Build history of the part. All positions in model axes, mm. A direction names the side the tool comes from. Coordinates: 2 decimals unless noted, no trailing zeros. Loops run counter-clockwise (first coordinate to the right, second up) from the corner with the lowest first, then second, coordinate; pieces in that order, holes last.
Item 1: 3-axis set-ups, long thin cutter, end or side, ignore diameter. For faces 1 (the face through (-32.5, 1, -71)), 2 (the face through (32.5, 1, -4)), 3 (the face through (-18, 2, 76)), 4 (the face through (32.5, 1, -71)): which of +Z, -Z, +X, -X, +Y, -Y reach the whole face in a straight line?
Item 2: Flat gauge pins, fed straight in: pin 1 (0.9 mm diameter, centred on y = 1, z = 60, fed in from -X); pin 2 (1.5 mm diameter, centred on x = 28, y = 1, fed in from +Z); pin 3 (0.8 mm diameter, centred on x = -33, y = 1, fed in from -Z). Where does each tip first touch, or does it go through?
Item 3: Drill centre lines: line 1 along Z through (x, y) = (-15.5, 1.9); line 2 along Y through (x, z) = (-3, -30.5); line 3 along X through (y, z) = (1.4, -46). Where is each one in solid material? Low to high.
Item 4: Cut at B-B (z = -51.5). List the corners of the cut face in (x, y), and give its area (3 significant figures).
Item 5: Mould opens along Z. For faces 5 (the face through (29, 2, 76)), 6 (the face through (-32.5, 1, -4)), 7 (the face through (-1, 0, 1)) say: released by +Z, released by -Z, zero draft, split by the parting line, or undercut.
from build123d import *

# Parameters (mm, degrees)
CROQUIS1_W               = 65
CROQUIS1_H               = 146
SALIENTE_EXTRUIR1_DEPTH  = 3
CROQUIS2_W               = 8
CROQUIS2_H               = 3
SALIENTE_EXTRUIR2_DEPTH  = 5
REDONDEO1_R              = 4
REDONDEO1_OF_SIMETR_A1_R = 4
CROQUIS3_W               = 2.60095456
CROQUIS3_H               = 3.001101416
SALIENTE_EXTRUIR3_DEPTH  = 0.8
REDONDEO2_R              = 2
REDONDEO2_OF_SIMETR_A5_R = 2
CROQUIS4_W               = 65
CROQUIS4_H               = 3
CROQUIS4_W_2             = 30
CROQUIS4_H_2             = 2
SALIENTE_EXTRUIR4_DEPTH  = 3
REDONDEO3_R              = 60


# Some blends are built 0.0001 mm under size
with BuildPart() as part:
    # Croquis1 → Saliente-Extruir1 (new body)
    with BuildSketch(Plane(origin=(0, 0, 0), x_dir=(1, 0, 0), z_dir=(0, 1, 0))):
        Rectangle(CROQUIS1_W, CROQUIS1_H)
    extrude(amount=SALIENTE_EXTRUIR1_DEPTH)

    # Croquis2 → Saliente-Extruir2 (add)
    with BuildSketch(Plane(origin=(32.5, 0, 0), x_dir=(0, 0, -1), z_dir=(1, 0, 0))):
        with Locations((66, 1.5)):
            Rectangle(CROQUIS2_W, CROQUIS2_H)
    saliente_extruir2 = extrude(amount=SALIENTE_EXTRUIR2_DEPTH)

    # Redondeo1
    redondeo1_edges = [part.edges().sort_by_distance(p)[0] for p in [
        (37.5, 1.5, -62),
        (37.5, 1.5, -70),
    ]]
    fillet(redondeo1_edges, radius=REDONDEO1_R - 0.0001)  # a hair under: the kernel refuses the full size

    # Simetría1: Saliente-Extruir2 across plane
    add(saliente_extruir2.mirror(Plane(origin=(0, 0, 0), x_dir=(0, 0, 1), z_dir=(1, 0, 0))))

    # Redondeo1 of Simetría1
    redondeo1_of_simetr_a1_edges = [part.edges().sort_by_distance(p)[0] for p in [
        (-37.5, 1.5, -62),
        (-37.5, 1.5, -70),
    ]]
    fillet(redondeo1_of_simetr_a1_edges, radius=REDONDEO1_OF_SIMETR_A1_R - 0.0001)  # a hair under: the kernel refuses the full size

    # Croquis3 → Saliente-Extruir3 (add)
    with BuildSketch(Plane(origin=(32.5, 0, 0), x_dir=(0, 0, -1), z_dir=(1, 0, 0))):
        with Locations((-53.003039433, 1.500550708)):
            Rectangle(CROQUIS3_W, CROQUIS3_H)
    saliente_extruir3 = extrude(amount=SALIENTE_EXTRUIR3_DEPTH)

    # Redondeo2
    # the kernel refuses this fillet: 2 mm, written as the material it takes off along each edge
    with BuildSketch(Plane(origin=(33.3, 7.001101416, 51.702562153), x_dir=(-1, 0, 0), z_dir=(0, -1, 0)), Plane(origin=(33.3, -4, 54.303516713), x_dir=(-1, 0, 0), z_dir=(0, 1, 0))) as redondeo2_piece_1:
        with BuildLine():
            CenterArc((2, -1.6), REDONDEO2_R, 126.869897646, 53.130102354)
            Line((0, -1.6), (-0.04, -1.6))
            Line((-0.04, -1.6), (-0.04, 0))
            Line((-0.04, 0), (0, 0.04))
            ThreePointArc((0, 0.04), (0.4, 0.04), (0.776, 0.032))
            Line((0.776, 0.032), (0.8, 0))
        make_face()
    extrude(amount=11.001101416, mode=Mode.SUBTRACT)

    # Simetría5: Saliente-Extruir3 across plane
    add(saliente_extruir3.mirror(Plane(origin=(0, 0, 0), x_dir=(0, 0, 1), z_dir=(1, 0, 0))))

    # Redondeo2 of Simetría5
    # the kernel refuses this fillet: 2 mm, written as the material it takes off along each edge
    with BuildSketch(Plane(origin=(-33.3, 7.001101416, 51.702562153), x_dir=(1, 0, 0), z_dir=(0, -1, 0)), Plane(origin=(-33.3, -4, 54.303516713), x_dir=(1, 0, 0), z_dir=(0, 1, 0))) as redondeo2_of_simetr_a5_piece_1:
        with BuildLine():
            CenterArc((2, 1.6), REDONDEO2_OF_SIMETR_A5_R, 180, 53.130102354)
            Line((0, 1.6), (-0.04, 1.6))
            Line((-0.04, 1.6), (-0.04, 0))
            Line((-0.04, 0), (0, -0.04))
            ThreePointArc((0, -0.04), (0.4, -0.04), (0.776, -0.032))
            Line((0.776, -0.032), (0.8, 0))
        make_face()
    extrude(amount=11.001101416, mode=Mode.SUBTRACT)

    # Croquis4 → Saliente-Extruir4 (add)
    with BuildSketch(Plane(origin=(0, 3, 0), x_dir=(1, 0, 0), z_dir=(0, 1, 0))):
        with Locations((0, -74.5)):
            Rectangle(CROQUIS4_W, CROQUIS4_H)
        with Locations((11.5, -77)):
            Rectangle(CROQUIS4_W_2, CROQUIS4_H_2)
    extrude(amount=-SALIENTE_EXTRUIR4_DEPTH)

    # Redondeo3
    # the kernel refuses this fillet: 60 mm, written as the material it takes off along each edge
    with BuildSketch(Plane(origin=(26.5, 41.405728739, 78), x_dir=(0, 0, -1), z_dir=(0, -1, 0))) as redondeo3_piece_1:
        with BuildLine():
            CenterArc((60, -15.362291496), REDONDEO3_R, 165.164888418, 14.835111582)
            Line((0, -15.362291496), (0, 0))
            Line((0, 0), (2, 0))
        make_face()
    extrude(amount=79.811457479, mode=Mode.SUBTRACT)
    with BuildSketch(Plane(origin=(-3.5, 41.405728739, 78), x_dir=(1, 0, 0), z_dir=(0, -1, 0))) as redondeo3_piece_2:
        with BuildLine():
            CenterArc((15.362291496, -60), REDONDEO3_R, 90, 14.835111582)
            Line((0, -2), (0, 0))
            Line((0, 0), (15.362291496, 0))
        make_face()
    extrude(amount=79.811457479, mode=Mode.SUBTRACT)


solid = part.part
Filled sheet:
1. face 1: -Z, -X, +Y, -Y
1. face 2: +X, +Y, -Y
1. face 3: +Z, -X, +Y, -Y
1. face 4: -Z, +X, +Y, -Y
2. pin 1: stops at x = -32.5
2. pin 2: stops at z = 76
2. pin 3: stops at z = -70
3. line 1: z = -73 to 76
3. line 2: y = 0 to 3
3. line 3: x = -32.5 to 32.5
4. outline: (-32.5, 0) - (32.5, 0) - (32.5, 3) - (-32.5, 3) - close
4. area: 195 mm2
5. face 5: released by +Z
5. face 6: undercut
5. face 7: zero draft
